Could you check a few things on this model? Use its own coordinates, in mm. Face numbers are marked on the shaded views. Coordinates: 2 decimals unless noted, no trailing zeros. Order: outer loops, then holes, each group sorted by start corner. A loop starts at its lowest first (then second) coordinate and runs counter-clockwise, first axis right, second up. Notation, with made-up numbers: (6.25, 65.5) -> (54.25, 65.5) arc R20 ccw to (54.25, 100.5) -> close; hole circle Ø4 at (-9.75, -9). An arc over 180 degrees is marked (long way). Put each result on its own line as item: value. Start each with the question number.
Q1. If we section it at C-C (x = 12.5): Please give me the cut outline in (y, z), and give its area (3 significant figures).
Q2. If we section it at A-A (z = 11): Please give me the cut outline in (x, y).
Q3. We'd pull the mould along Z, two halves only. Please class the marked faces 1, 2, 3 and 4: +Z half, -Z half, draft (parallel to the pull), parting line (faces both ways), or undercut.
Q4. If we section it at B-B (x = -10): Please give me the cut outline in (y, z), and give its area (3 significant figures).
Q5. Will these pins go through, and if not, where does the flat tip stop? pin 1 (12 mm diameter, centred on x = 3.5, z = -9.5, fed in from +Y); pin 2 (4 mm diameter, centred on y = 13.5, z = -1.5, fed in from -X).
Q6. Please list where these lines run through material, in increasing order: line 1 along X through (y, z) = (1.2, -10); line 2 along X through (y, z) = (1.2, 10); line 3 along Y through (x, z) = (-9, -1.5).
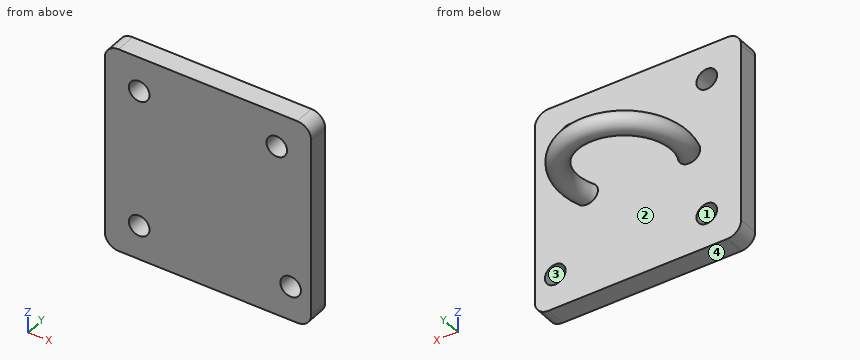
from build123d import *

# Parameters (mm, degrees)
SKETCH1_W           = 30
SKETCH1_H           = 30
BOSS_EXTRUDE1_DEPTH = 3
SWEEP1_PROFILE_R    = 1.5
SKETCH12_R          = 1.5
CUT_EXTRUDE1_DEPTH  = 3
FILLET1_R           = 2


with BuildPart() as part:
    # Sketch1 → Boss-Extrude1 (new body)
    with BuildSketch(Plane(origin=(0, 0, 0), x_dir=(1, 0, 0), z_dir=(0, 1, 0))):
        Rectangle(SKETCH1_W, SKETCH1_H)
    extrude(amount=BOSS_EXTRUDE1_DEPTH)

    # Sweep1: sweep along a path in Sketch2
    with BuildLine(Plane.XY) as sweep1_path:
        ThreePointArc((6.607920582, 1.389009429), (0, 13.898486736), (-6.607920582, 1.389009429))
    # Sweep1 profile (on start of the path) → Sweep1 (sweep)
    with BuildSketch(Plane(origin=(6.607920582, 1.389009429, 0), x_dir=(0.8259900728012373, -0.5636846632948309, 0), z_dir=(0.5636846632948309, 0.8259900728012373, 0))):
        Circle(SWEEP1_PROFILE_R)
    sweep(path=sweep1_path.line)

    # Sketch12 → Cut-Extrude1 (cut)
    with BuildSketch(Plane(origin=(0, 3, 0), x_dir=(1, 0, 0), z_dir=(0, 1, 0))):
        with Locations(Location((-10, 10, 0), (0, 0, 270))):
            Circle(SKETCH12_R)
        with Locations(Location((12.019460679, 10, 0), (0, 0, 270))):
            Circle(SKETCH12_R)
        with Locations(Location((10, -10, 0), (0, 0, 270))):
            Circle(SKETCH12_R)
        with Locations(Location((-10, -10, 0), (0, 0, 270))):
            Circle(SKETCH12_R)
    extrude(amount=-CUT_EXTRUDE1_DEPTH, mode=Mode.SUBTRACT)

    # Fillet1
    fillet1_edges = [part.edges().sort_by_distance(p)[0] for p in [
        (15, 1.5, 15),
        (-15, 1.5, 15),
        (-15, 1.5, -15),
        (15, 1.5, -15),
    ]]
    fillet(fillet1_edges, radius=FILLET1_R)


solid = part.part
The answers:
1. outline: (0, -15) -> (3, -15) -> (3, -11.42) -> (0, -11.42) -> close; (0, -8.58) -> (3, -8.58) -> (3, 15) -> (0, 15) -> close
1. area: 81.5 mm^2
2. outline: (-15, 0) -> (-11.12, 0) -> (-11.12, 3) -> (-15, 3) -> close; (-8.88, 0) -> (8.88, 0) -> (8.88, 3) -> (-8.88, 3) -> close; (11.12, 0) -> (15, 0) -> (15, 3) -> (11.12, 3) -> close
3. face 1: undercut
3. face 2: draft
3. face 3: undercut
3. face 4: -Z half
4. outline: (0, -15) -> (3, -15) -> (3, -11.5) -> (0, -11.5) -> close; (0, -8.5) -> (3, -8.5) -> (3, 8.5) -> (0, 8.5) -> close; (0, 11.5) -> (3, 11.5) -> (3, 15) -> (0, 15) -> close
4. area: 72.0 mm^2
5. pin 1: y = 3
5. pin 2: x = -7.36
6. line 1: -15 to -11.5, -8.5 to 10.52, 13.52 to 15
6. line 2: -15 to -11.5, -8.5 to 8.5, 11.5 to 15
6. line 3: 0 to 3
